Design review of the part built by this model. Coordinates are the model's own, in mm. A direction names the side the tool comes from. Give positions to 0.01 mm unless a question says otherwise; leave off trailing zeros. Loops run counter-clockwise (first coordinate to the right, second up) from the corner with the lowest first, then second, coordinate; pieces in that order, holes last. Notation, with made-up numbers: (74.25, 78.25) - (84.25, 78.25) arc R19 ccw to (84.25, 88.25) - close; hole circle Ø7 at (28, -15). An arc over 180 degrees is marked (long way). Write each question's results on one line, items separated by ' | '.
```python
from build123d import *

# Parameters (mm, degrees)
SKETCH_1_R      = 35
EXTRUDE_1_DEPTH = 6


with BuildPart() as part:
    # 草图1 → 凸台-拉伸1 (new body)
    with BuildSketch(Plane(origin=(0, 0, 0), x_dir=(1, 0, 0), z_dir=(0, 1, 0))):
        with Locations(Location((0, 0, 0), (0, 0, 270))):
            Circle(SKETCH_1_R)
        with BuildLine():
            ThreePointArc((-20.982160881, 14.491339648), (-26.480889225, 16.592920354), (-22.19153101, 12.561287809))
            ThreePointArc((-22.19153101, 12.561287809), (-25.5, 0), (-22.19153101, -12.561287809))
            ThreePointArc((-22.19153101, -12.561287809), (-26.480889225, -16.592920354), (-20.982160881, -14.491339648))
            ThreePointArc((-20.982160881, -14.491339648), (7.04399237, -24.507798177), (25.474557522, -1.138823539))
            ThreePointArc((25.474557522, -1.138823539), (31.25, 0), (25.474557522, 1.138823539))
            ThreePointArc((25.474557522, 1.138823539), (7.04399237, 24.507798177), (-20.982160881, 14.491339648))
        make_face(mode=Mode.SUBTRACT)
    extrude(amount=EXTRUDE_1_DEPTH)


solid = part.part
```
Item 1: We need section C-C on y = 3.8. Give the boundary of the cut face in (x, z).
Output values:
outline: circle Ø70 at (0, 0); hole (-22.19, -12.56) arc R3 ccw (long way) to (-20.98, -14.49) arc R25.5 ccw to (25.47, -1.14) arc R3 ccw (long way) to (25.47, 1.14) arc R25.5 ccw to (-20.98, 14.49) arc R3 ccw (long way) to (-22.19, 12.56) arc R25.5 ccw to start
Item 2: Draft analysis for pull direction X (two halves, no side actions). For faces 3 (the face through (-26.418, 2.958, -16.69)), 4 (the face through (18.3, 0, 18)), 5 (the face through (-21, 3, -28)), state which applies: +X half, -X half, draft (parallel to the pull), parting line (faces both ways), or undercut.
Output values:
face 3: undercut | face 4: draft | face 5: parting line
Item 3: We need section A-A on z = 0. Give the boundary of the cut face in (x, y), then the cut area to 3 significant figures.
Output values:
outline: (-35, 0) - (-25.5, 0) - (-25.5, 6) - (-35, 6) - close; (31.25, 0) - (35, 0) - (35, 6) - (31.25, 6) - close | area: 79.5 mm²
Item 4: Tool access review of faces 1 (the face through (6.615, 2.958, 24.627)), 2 (the face through (18.3, 6, 18)): name each direction out of +Z, -Z, +X, -X, +Y, -Y from which nothing blocks a thin tool from reaching the whole face with its end or side.
Output values:
face 1: +Y, -Y | face 2: +Z, -Z, +X, -X, +Y
Item 5: We need section B-B on x = 29. Give the boundary of the cut face in (y, z).
Output values:
outline: (0, -19.6) - (6, -19.6) - (6, -2.9) - (0, -2.9) - close; (0, 2.9) - (6, 2.9) - (6, 19.6) - (0, 19.6) - close
Item 6: We need section D-D on z = -27. Give the boundary of the cut face in (x, y).
Output values:
outline: (-22.27, 0) - (22.27, 0) - (22.27, 6) - (-22.27, 6) - close
Item 7: Wall thickness on probe 1 along X at (y, z) = (2.3, -15); probe 2 along Z at (x, y) = (-22.5, 3.35); probe 3 along X at (y, z) = (0.9, 6.5): over which ranges is each line inside the solid? List them lowest first.
Output values:
probe 1: x = -31.62 to -26.94, -20.94 to -20.62, 20.62 to 31.62 | probe 2: z = -26.81 to -17.63, -12.37 to -12, 12 to 12.37, 17.63 to 26.81 | probe 3: x = -34.39 to -24.66, 24.66 to 34.39
Item 8: Clearance check with flat-ended pins moving along their axes: P1, Ø2, axis at x = 22.5, y = 3.5, coming from the -Z side; P2, Ø3.5, axis at x = -23.94, z = 15, coming from the +Y side; P3, Ø1, axis at y = 1.5, z = 26, coming from the -X side. State where each tip first meets the part, or that it passes through.
Output values:
P1: stops at z = -27.62 | P2: passes through | P3: stops at x = -23.97
